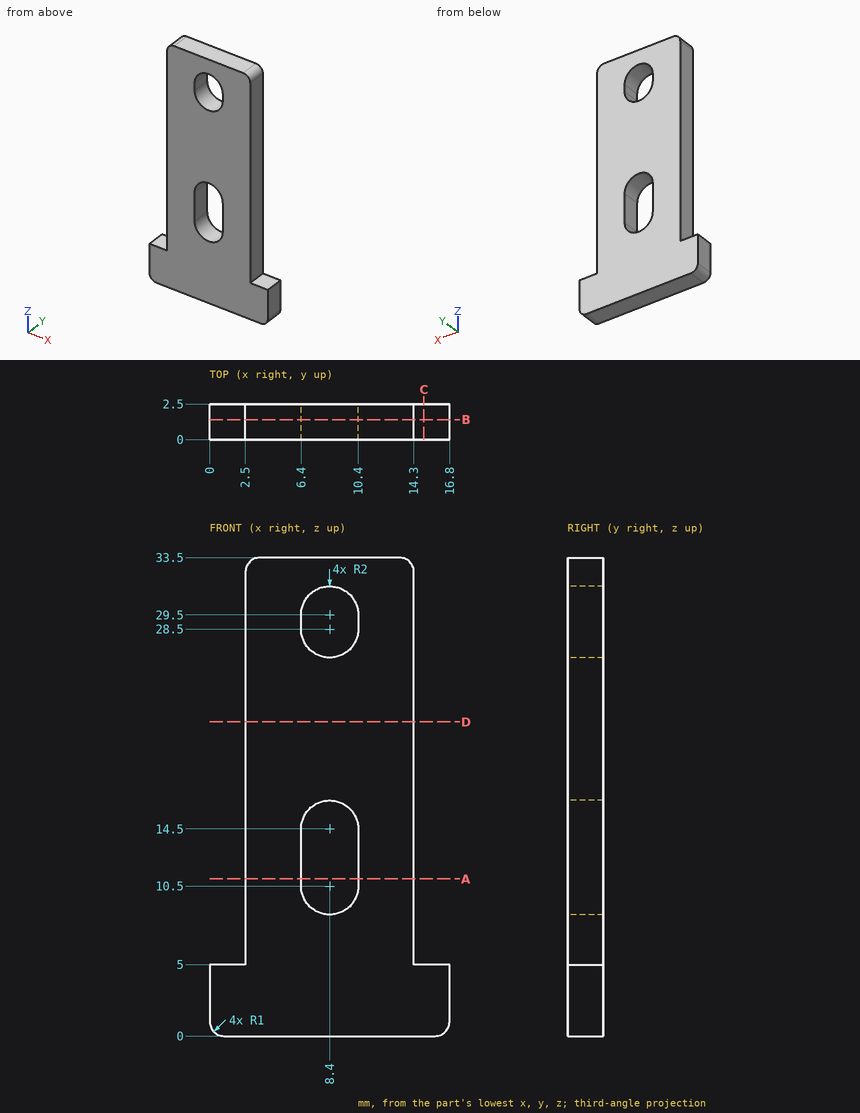
Here's the drawing with two shaded views (mm, measured from the low corner). I have some questions. Give positions to 0.01 mm unless a question says otherwise; leave off trailing zeros. Loops run counter-clockwise (first coordinate to the right, second up) from the corner with the lowest first, then second, coordinate; pieces in that order, holes last. Notation, with made-up numbers: (17, -2.5) -> (47, -2.5) arc R7 cw to (47, 4.5) -> close; hole circle Ø1 at (81.25, -16.5). An arc over 180 degrees is marked (long way). One line per item, written item: value.
Q1. Suppose I cut it at C-C on x = 15. Please give me the cut outline in (y, z), then the cut area to 3 significant figures.
Answers follow:
outline: (0, 0) -> (2.5, 0) -> (2.5, 5) -> (0, 5) -> close
area: 12.5 mm^2
Q2. Suppose I cut it at D-D on z = 22. Please give me the cut outline in (x, y), then the cut area to 3 significant figures.
Answers follow:
outline: (2.5, 0) -> (14.3, 0) -> (14.3, 2.5) -> (2.5, 2.5) -> close
area: 29.5 mm^2
Q3. I'm going to push flat-ended pins straight in: pin 1 Ø0.5 at (y, z) = (1.5, 29) entering from +X; pin 2 Ø1.2 at (x, y) = (1, 1.5) entering from +Z; pin 3 Ø1.1 at (y, z) = (1.5, 29) entering from -X. Where does each tip first touch, or does it pass through?
Answers follow:
pin 1: x = 14.3
pin 2: z = 5
pin 3: x = 2.5
Q4. Suppose I cut it at A-A on z = 11. Please give me the cut outline in (x, y).
Answers follow:
outline: (2.5, 0) -> (6.4, 0) -> (6.4, 2.5) -> (2.5, 2.5) -> close; (10.4, 0) -> (14.3, 0) -> (14.3, 2.5) -> (10.4, 2.5) -> close
Q5. Suppose I cut it at B-B on y = 1.4. Please give me the cut outline in (x, z).
Answers follow:
outline: (0, 1) arc R1 ccw to (1, 0) -> (15.8, 0) arc R1 ccw to (16.8, 1) -> (16.8, 5) -> (14.3, 5) -> (14.3, 32.5) arc R1 ccw to (13.3, 33.5) -> (3.5, 33.5) arc R1 ccw to (2.5, 32.5) -> (2.5, 5) -> (0, 5) -> close; hole (6.4, 10.5) arc R2 ccw to (10.4, 10.5) -> (10.4, 14.5) arc R2 ccw to (6.4, 14.5) -> close; hole (6.4, 28.5) arc R2 ccw to (10.4, 28.5) -> (10.4, 29.5) arc R2 ccw to (6.4, 29.5) -> close
Q6. If I drill on line 1 along X through (y, z) = (0.15, 14); line 2 along Z through (x, y) = (6.75, 0.3); line 3 along Z through (x, y) = (9.75, 0.55), over which ranges is the centre line in solid material (lowest first)?
Answers follow:
line 1: 2.5 to 6.4, 10.4 to 14.3
line 2: 0 to 9.37, 15.63 to 27.37, 30.63 to 33.5
line 3: 0 to 9.02, 15.98 to 27.02, 30.98 to 33.5
